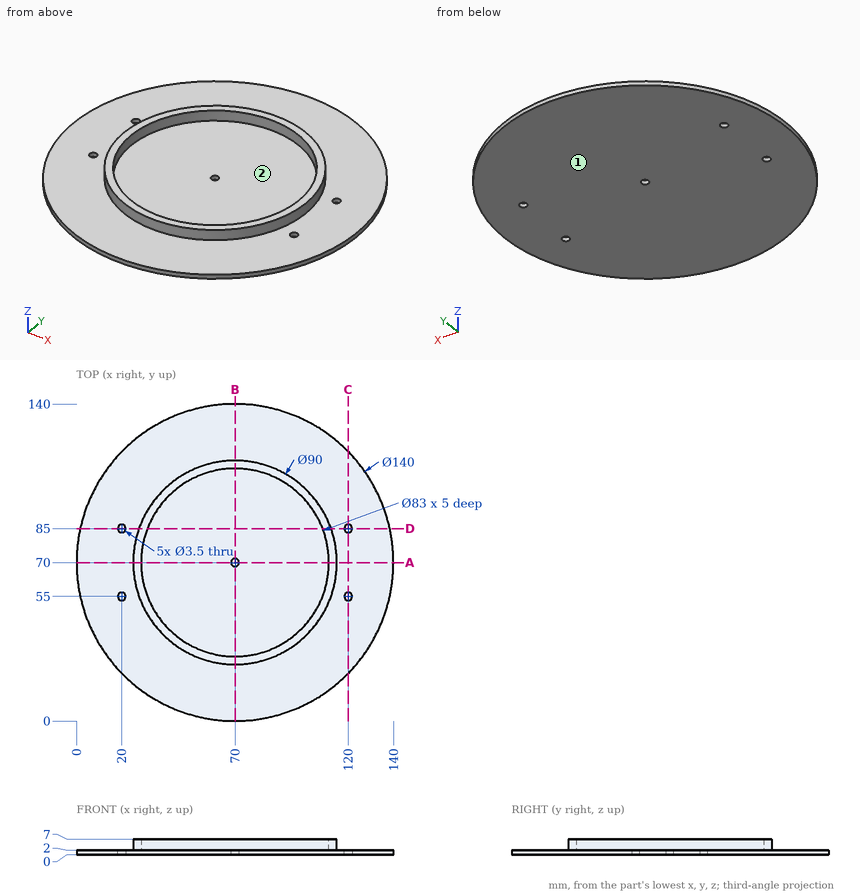
Source: three-view drawing plus pictorial views. Frame: mm from the lowest corner of the part. Give positions to 0.01 mm unless a question says otherwise; leave off trailing zeros. Loops run counter-clockwise (first coordinate to the right, second up) from the corner with the lowest first, then second, coordinate; pieces in that order, holes last. Notation, with made-up numbers: (43, 40.25) -> (52, 40.25) arc R22 cw to (52, 78.25) -> close; hole circle Ø4 at (58, 6.25). An arc over 180 degrees is marked (long way). Use a Markdown table: item, result. Add a question column.
(1) First-contact query: pin 1 Ø4.5 at (x, y) = (120, 85) entering from +Z; pin 2 Ø3 at (x, z) = (31.5, 3) entering from +Y; pin 3 Ø1.5 at (x, z) = (116.5, 1.5) entering from +Y. Flat tips, straight axial feed; report the tip coordinate or a pass-through.
(2) Pull-direction query (Y, two-part tool) for the marked faces 1 and 2; classes: +Y half, -Y half, draft (parallel to the pull), parting line (faces both ways), or undercut.
(3) Section query A-A (y = 70). Output: boundary loops of the cut face in (x, z), then the cut area to 3 significant figures.
(4) Section query D-D (y = 85). Output: boundary loops of the cut face in (x, z).
(5) Section query C-C (x = 120). Output: boundary loops of the cut face in (y, z).
(6) Ray query, line 1 (Y direction, x = 20, z = 1.25); line 2 (Y direction, x = 70, z = 4.05); line 3 (X direction, y = 85, z = 0.5). Return the intervals inside material, ascending.
Checked values:
| question | item | result |
|---|---|---|
| 1 | pin 1 | z = 2 |
| 1 | pin 2 | y = 129.18 |
| 1 | pin 3 | y = 122.98 |
| 2 | face 1 | draft |
| 2 | face 2 | undercut |
| 3 | outline | (0, 0) -> (68.25, 0) -> (68.25, 2) -> (28.5, 2) -> (28.5, 7) -> (25, 7) -> (25, 2) -> (0, 2) -> close; (71.75, 0) -> (140, 0) -> (140, 2) -> (115, 2) -> (115, 7) -> (111.5, 7) -> (111.5, 2) -> (71.75, 2) -> close |
| 3 | area | 308 mm^2 |
| 4 | outline | (1.63, 0) -> (18.25, 0) -> (18.25, 2) -> (1.63, 2) -> close; (21.75, 0) -> (118.25, 0) -> (118.25, 2) -> (112.43, 2) -> (112.43, 7) -> (108.69, 7) -> (108.69, 2) -> (31.31, 2) -> (31.31, 7) -> (27.57, 7) -> (27.57, 2) -> (21.75, 2) -> close; (121.75, 0) -> (138.37, 0) -> (138.37, 2) -> (121.75, 2) -> close |
| 5 | outline | (21.01, 0) -> (53.25, 0) -> (53.25, 2) -> (21.01, 2) -> close; (56.75, 0) -> (83.25, 0) -> (83.25, 2) -> (56.75, 2) -> close; (86.75, 0) -> (118.99, 0) -> (118.99, 2) -> (86.75, 2) -> close |
| 6 | line 1 | 21.01 to 53.25, 56.75 to 83.25, 86.75 to 118.99 |
| 6 | line 2 | 25 to 28.5, 111.5 to 115 |
| 6 | line 3 | 1.63 to 18.25, 21.75 to 118.25, 121.75 to 138.37 |
